Input: part model. Units: mm. Frame: model coordinates. A direction names the side the tool comes from. Coordinates: 2 decimals unless noted, no trailing zeros. Loops run counter-clockwise (first coordinate to the right, second up) from the corner with the lowest first, then second, coordinate; pieces in that order, holes last.
(1) Line query: L1, parallel to Y at x = 0, z = 17.75; L2, parallel to Y at x = 5, z = 30.5. Output: solid intervals per line, ascending.
(2) Section A-A, the plane z = 9.5. Return loops of the section in (x, y).
(3) Mould query, pull axis X, two halves, no side actions, for faces 3 (the face through (-0.676, 3.044, 15.835)), 4 (the face through (-2.17, 9.76, 0.7)), 5 (the face through (0, 0, 0)). Classes: released by +X, released by -X, zero draft, split by the parting line, or undercut.
(4) Contact query for flat-ended pins moving along their axis: P1, Ø2, axis at x = 7.5, z = 37.5, coming from the +Y side; P2, Ø9.5, axis at x = 2.5, y = -4.5, coming from the +Z side; P3, Ø10, axis at y = 7.5, z = 33.5, coming from the +X side. Output: stop coordinate, or through.
(5) Set-up query: faces 1 (the face through (0, 0, 8.892)), 2 (the face through (-2, -2, 7.972)). Return all of +Z, -Z, +X, -X, +Y, -Y with unobstructed straight access to the full face (end or side cutting, diameter ignored); none if empty.
```python
from build123d import *

# Parameters (mm, degrees)
F2_R = 0.5


# Not quite as in the source:
# - a feature of the source that left no trace in its solid (it failed there, or was rolled back) is left out
# - the dataset's text gives a spline's control points without its knots; the knots are read off the source's solid


with BuildPart() as f1:
    # F0 (on Front) → F1 (revolve)
    with BuildSketch(Plane.XZ):
        with BuildLine():
            Line((0, 8.8922893628), (0, 0))
            Line((0, 0), (10, 0))
            Line((10, 0), (10, 1.8884923775))
            Line((10, 1.8884923775), (1.8822399434, 1.8884923775))
            Line((1.8822399434, 1.8884923775), (1.8822399434, 7.9723326489))
            Line((1.8822399434, 7.9723326489), (3.9016692663, 7.9723326489))
            Line((3.9016692663, 7.9723326489), (3.9016692663, 22.0649164012))
            add(Edge.make_bspline(
                [(3.9016692663, 22.0649164012), (5.1630344119, 23.1520306668), (8.0559152247, 25.6452753955), (16.5026077823, 29.9379306564), (12.263488456, 50.8664231488), (12.3197676064, 51.0582432728), (12.3233571649, 51.0704778135)],
                knots=[0, 0, 0, 0, 0.2311293716, 0.5300841921, 0.9700281494, 1, 1, 1, 1], degree=3))
            Line((12.3233571649, 51.0704778135), (11.1718934655, 51.4083120162))
            add(Edge.make_bspline(
                [(3.1182529682, 22.9739045768), (3.4593403907, 23.2678725877), (4.1477996012, 23.8612916433), (5.055986388, 24.612670911), (5.8294364602, 25.2158290825), (6.4375839903, 25.6679744102), (7.0775050494, 26.1193928261), (7.7560186195, 26.5667311764), (8.4251192748, 26.9969284999), (9.2952385489, 27.5836159192), (10.3082664571, 28.3821097797), (11.1679720476, 29.3787760328), (11.7453344155, 30.3863434128), (12.1149836837, 31.2792473003), (12.4063741535, 32.3328106346), (12.6064087785, 33.5969680598), (12.7182156401, 35.0371100675), (12.7583513738, 37.1240288557), (12.6305002665, 39.940511974), (12.3457983074, 42.7678000329), (12.0752385257, 44.8846941108), (11.8638140518, 46.3626203182), (11.656802466, 47.6938398023), (11.4987113533, 48.6504829476), (11.3872612278, 49.3063855837), (11.3127390143, 49.7393978893), (11.2487872649, 50.1095476693), (11.196769712, 50.4138822278), (11.1642496864, 50.6115467989), (11.1446042442, 50.7412492276), (11.1324663607, 50.8302814164), (11.1222249941, 50.9294704016), (11.1171182056, 51.0396395949), (11.1237031708, 51.1661769089), (11.1386792065, 51.2763017797), (11.1621810328, 51.3767208912), (11.1714256361, 51.4067174809), (11.1718934655, 51.4083120162)],
                knots=[1.1e-09, 1.1e-09, 1.1e-09, 1.1e-09, 0.0625, 0.125, 0.15625, 0.1875, 0.21875, 0.25, 0.28125, 0.3125, 0.375, 0.4375, 0.46875, 0.5, 0.53125, 0.5625, 0.59375, 0.625, 0.6875, 0.75, 0.78125, 0.8125, 0.84375, 0.875, 0.890625, 0.90625, 0.921875, 0.9375, 0.953125, 0.9609375, 0.96875, 0.9765625, 0.984375, 0.98828125, 0.9921875, 0.99609375, 1, 1, 1, 1], degree=3))
            Line((3.1182529682, 22.9739045768), (3.1182529682, 8.8922893628))
            Line((3.1182529682, 8.8922893628), (1.4163269661, 8.8922893628))
            Line((1.4163269661, 8.8922893628), (0, 8.8922893628))
        make_face()
    revolve(axis=Axis((0, 0, 4.4461446814), (0, 0, -1)))

    # F2
    f2_edges = [f1.edges().sort_by_distance(p)[0] for p in [
        (-1.88224, 0, 1.888492),
        (-1.88224, 0, 7.972333),
        (1.88224, 0, 4.930413),
        (-10, 0, 1.888492),
    ]]
    fillet(f2_edges, radius=F2_R)


solid = f1.part
```
Report:
1. L1: y = -3.9 to -3.12, 3.12 to 3.9
1. L2: y = -12.09 to -10.66, 10.66 to 12.09
2. outline: circle Ø7.8 at (0, 0); hole circle Ø6.24 at (0, 0)
3. face 3: undercut
3. face 4: split by the parting line
3. face 5: zero draft
4. P1: stops at y = 12.31
4. P2: stops at z = 28.08
4. P3: stops at x = 13.63
5. face 1: +Z
5. face 2: none
